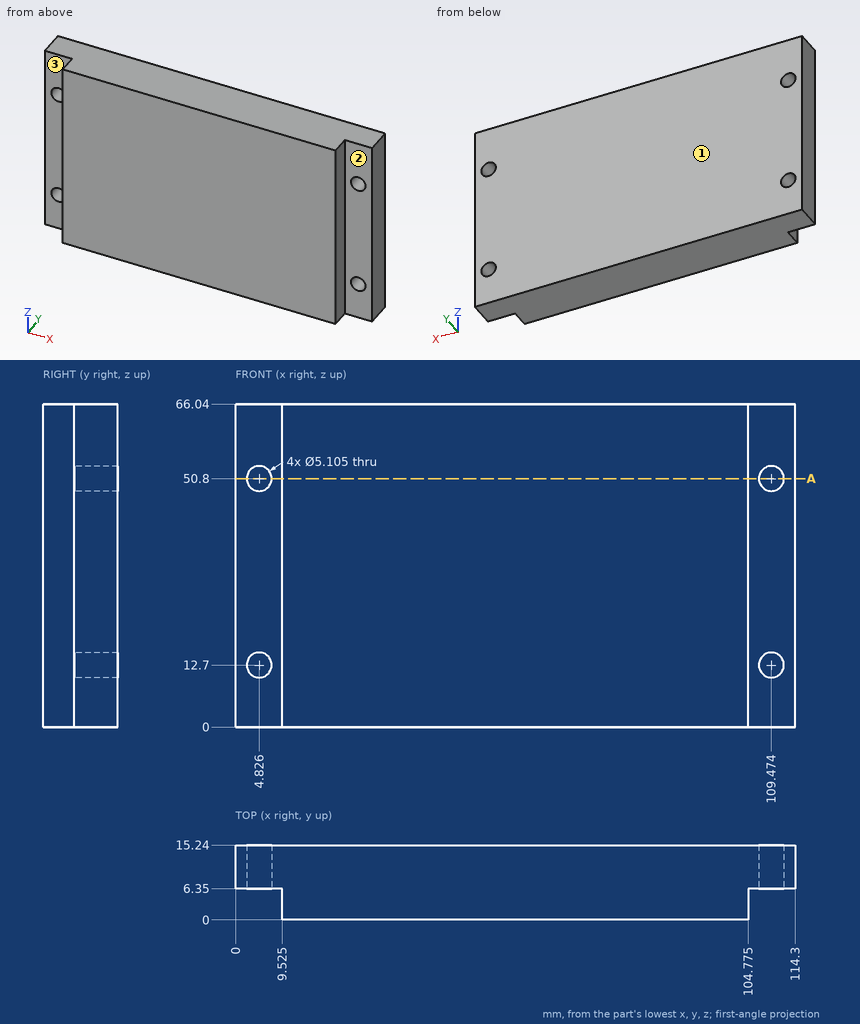
Check sheet for the drawn part. Datum: minimum x, y, z corner. Units: mm. A direction names the side the tool comes from. Coordinates: 2 decimals unless noted, no trailing zeros. Answer in a Markdown table with one row per item.
1. Sectioned sample at A-A, the plane z = 50.8. Give the number of separate pieces and of enclosed holes in the cut face, then the cut area to 3 significant figures.
Check values:
| item | result |
|---|---|
| separate pieces | 3 |
| enclosed holes | 0 |
| area | 1,530 mm2 |
2. Material ranges on line 1 along X through (y, z) = (12, 12.7); line 2 along Z through (x, y) = (5.5, 6.75); line 3 along X through (y, z) = (9, 13.5), recorded low to high. Write a range as [from, to].
Check values:
| item | result |
|---|---|
| line 1 | x = [0, 2.27], [7.38, 106.92], [112.03, 114.3] |
| line 2 | z = [0, 10.24], [15.16, 48.34], [53.26, 66.04] |
| line 3 | x = [0, 2.4], [7.25, 107.05], [111.9, 114.3] |
3. Access from +Z, -Z, +X, -X, +Y, -Y to the whole of each face (thin tool, end or side, straight path). Record for the marked faces 1, 2 and 3.
Check values:
| item | result |
|---|---|
| face 1 | +Z, -Z, +X, -X, +Y |
| face 2 | +Z, -Z, +X, -Y |
| face 3 | +Z, -Z, -X, -Y |
4. Go/stop test with flat-tipped pins: pin 1 (3 mm diameter, centred on x = 2.5, z = 26.5, fed in from -Y); pin 2 (3 mm diameter, centred on y = 2.5, z = 44.5, fed in from +X) (3 decimals). Record where each tip stops, or that it passes through.
Check values:
| item | result |
|---|---|
| pin 1 | stops at y = 6.35 |
| pin 2 | stops at x = 104.775 |
